```python
from build123d import *

# Parameters (mm, degrees)
SKETCH_2_W          = 30
SKETCH_2_H          = 60
SKETCH_2_W_2        = 20
SKETCH_2_H_2        = 40
EXTRUDE_1_DEPTH     = 5
SKETCH_3_R          = 2
CUT_EXTRUDE_1_DEPTH = 5
EXTRUDE_2_DEPTH     = 5
SKETCH_6_R          = 1.5
CUT_EXTRUDE_2_DEPTH = 5


with BuildPart() as part:
    # 草图2 → 凸台-拉伸1 (new body)
    with BuildSketch(Plane.XY):
        with Locations((10, -20)):
            Rectangle(SKETCH_2_W, SKETCH_2_H)
        with Locations((10, -20)):
            Rectangle(SKETCH_2_W_2, SKETCH_2_H_2, mode=Mode.SUBTRACT)
    extrude(amount=EXTRUDE_1_DEPTH)

    # 草图3 → 切除-拉伸1 (cut)
    with BuildSketch(Plane.XY.offset(5)):
        with Locations((15.25, 5.5)):
            Circle(SKETCH_3_R)
        with Locations((15.25, -45.5)):
            Circle(SKETCH_3_R)
        with Locations((4.75, -45.5)):
            Circle(SKETCH_3_R)
        with Locations((4.75, 5.5)):
            Circle(SKETCH_3_R)
    extrude(amount=-CUT_EXTRUDE_1_DEPTH, mode=Mode.SUBTRACT)

    # 草图5 → 凸台-拉伸2 (add)
    with BuildSketch(Plane(origin=(25, 0, 0), x_dir=(0, 0, -1), z_dir=(1, 0, 0))):
        with BuildLine():
            Line((-5, -42), (-5, -40))
            Line((-5, -40), (0, -40))
            Line((0, -40), (0, -42))
            ThreePointArc((0, -42), (0.878679656, -44.121320344), (3, -45))
            Line((3, -45), (20, -45))
            Line((20, -45), (20, -50))
            Line((20, -50), (0, -50))
            Line((0, -50), (-5, -50))
            Line((-5, -50), (-25, -50))
            Line((-25, -50), (-25, -45))
            Line((-25, -45), (-8, -45))
            ThreePointArc((-8, -45), (-5.878679656, -44.121320344), (-5, -42))
        make_face()
    extrude_2 = extrude(amount=EXTRUDE_2_DEPTH)

    # 镜向1: 凸台-拉伸2 across plane
    add(extrude_2.mirror(Plane(origin=(10, 0, 0), x_dir=(0, 0, 1), z_dir=(1, 0, 0))))

    # 草图6 → 切除-拉伸2 (cut)
    with BuildSketch(Plane(origin=(0, -45, 0), x_dir=(1, 0, 0), z_dir=(0, 1, 0))):
        with Locations(Location((-7.5, 12.5, 0), (0, 0, 270))):
            Circle(SKETCH_6_R)
        with Locations(Location((-7.5, -17.5, 0), (0, 0, 270))):
            Circle(SKETCH_6_R)
        with Locations(Location((27.5, -17.5, 0), (0, 0, 270))):
            Circle(SKETCH_6_R)
        with Locations(Location((27.5, 12.5, 0), (0, 0, 270))):
            Circle(SKETCH_6_R)
    extrude(amount=-CUT_EXTRUDE_2_DEPTH, mode=Mode.SUBTRACT)


solid = part.part
```
The listing builds one solid part. Answer for the finished solid, in the listing's coordinates (mm). A direction names the side the tool comes from. Coordinates: 2 decimals unless noted, no trailing zeros. Loops run counter-clockwise (first coordinate to the right, second up) from the corner with the lowest first, then second, coordinate; pieces in that order, holes last. Notation, with made-up numbers: (10.5, 46) - (27.5, 46) arc R7 ccw to (27.5, 58) - close; hole circle Ø7 at (79.5, 66). An arc over 180 degrees is marked (long way). Write item = value, one per line.
1) Determine the mould class of faces 1 (the face through (-7.43, -47.46, 16)), 2 (the face through (30, -47, 2)), 3 (the face through (-7, -48, 25)) for opening direction X: pulls with the +X half, pulls with the -X half, needs draft (parallel to the pull), parting line crosses it, or undercut.
Responses:
face_1 = undercut
face_2 = pulls with the +X half
face_3 = needs draft
2) Section D-D (x = 27.5) is taken. Determine the outline of the cut face in (y, z), plus the area to 3 significant figures.
Responses:
outline = (-50, -20) - (-45, -20) - (-45, -14) - (-50, -14) - close; (-50, -11) - (-45, -11) - (-45, -3) arc R3 cw to (-42, 0) - (-40, 0) - (-40, 5) - (-42, 5) arc R3 cw to (-45, 8) - (-45, 16) - (-50, 16) - close; (-50, 19) - (-45, 19) - (-45, 25) - (-50, 25) - close
area = 224 mm^2
3) Section C-C (y = -26.5) is taken. Determine the outline of the cut face in (x, z).
Responses:
outline = (-5, 0) - (0, 0) - (0, 5) - (-5, 5) - close; (20, 0) - (25, 0) - (25, 5) - (20, 5) - close
4) Section B-B (x = 12.5) is taken. Determine the outline of the cut face in (y, z), plus the area to 3 significant figures.
Responses:
outline = (-50, 0) - (-40, 0) - (-40, 5) - (-50, 5) - close; (0, 0) - (10, 0) - (10, 5) - (0, 5) - close
area = 100 mm^2
5) Section A-A (z = 17.5) is taken. Determine the outline of the cut face in (x, y), plus the area to 3 significant figures.
Responses:
outline = (-10, -50) - (-9, -50) - (-9, -45) - (-10, -45) - close; (-6, -50) - (-5, -50) - (-5, -45) - (-6, -45) - close; (25, -50) - (26, -50) - (26, -45) - (25, -45) - close; (29, -50) - (30, -50) - (30, -45) - (29, -45) - close
area = 20.0 mm^2
6) Each of these flat-tipped pins is pushed along its axis until it touches: P1, Ø5.5, axis at x = 28.5, z = -12, coming from the +Y side; P2, Ø1.8, axis at x = -7.5, z = -12.5, coming from the +Y side; P3, Ø1.5, axis at y = -29.5, z = 2, coming from the +X side; P4, Ø10, axis at x = 17, y = 0, coming from the -Z side. Where does it stop, or does it pass through?
Responses:
P1 = -45
P2 = through
P3 = 25
P4 = 0
7) Find the intervals of material crossed by line 1 along X through (y, z) = (-46.05, 17.5); line 2 along Y through (x, z) = (15.25, 3.3); line 3 along Z through (x, y) = (27, -46), in increasing order.
Responses:
line_1 = -10 to -9, -6 to -5, 25 to 26, 29 to 30
line_2 = -50 to -47.5, -43.5 to -40, 0 to 3.5, 7.5 to 10
line_3 = -20 to -13.91, -11.09 to 16.09, 18.91 to 25
8) Which of the six approach directions +Z, -Z, +X, -X, +Y, -Y give full straight-line access (tool end or side, diameter ignored) to faces 4 (the face through (-5.8, -45, 16.6)), 5 (the face through (27, -40, 3)), 6 (the face through (20, -20, 2)), 7 (the face through (-9, -45, -11)), 8 (the face through (-7, -40, 3))?
Responses:
face_4 = +Z, +X, -X, +Y
face_5 = +Z, -Z, +X, +Y
face_6 = +Z, -Z
face_7 = -Z, +X, -X, +Y
face_8 = +Z, -Z, -X, +Y
